Could you check a few things on this model? Use its own coordinates, in mm. Face numbers are marked on the shaded views. A direction names the side the tool comes from. Give positions to 0.01 mm unless a question says otherwise; leave off trailing zeros. Order: outer loops, then holes, each group sorted by start corner. A loop starts at its lowest first (then second) coordinate and runs counter-clockwise, first axis right, second up. Notation, with made-up numbers: M 10.25,70.5 L 39.25,70.5 A7 ccw 39.25,83.5 Z; hole C -5,60 d3. An arc over 180 degrees is marked long. Use a Markdown table: item, result. Add a question column.
```python
from build123d import *

# Parameters (mm, degrees)
F1_DEPTH = 21.59
F2_R     = 4.7625
F3_DEPTH = 25.4
F4_R     = 6.35
F5_DEPTH = 25.4
F6_R     = 10.16


with BuildPart() as f1:
    # F0 (on Top) → F1 (new body)
    with BuildSketch(Plane.XY):
        Polygon((53.34, 0), (0, 0), (-53.34, 0), (-65.4083, -34.193517), (-70.758128, -34.193517), (-68.58, -43.18), (-53.34, -43.18), (-43.478824, -15.24), (0, -15.24), (43.478824, -15.24), (53.34, -43.18), (68.58, -43.18), (70.758128, -34.193517), (65.4083, -34.193517), align=None)
    extrude(amount=F1_DEPTH)

    # F2 (on face) → F3 (cut)
    with BuildSketch(Plane.XZ.offset(43.18)):
        with Locations((-60.96, 10.795)):
            Circle(F2_R)
        with Locations((60.96, 10.795)):
            Circle(F2_R)
    extrude(amount=-F3_DEPTH, mode=Mode.SUBTRACT)

    # F4 (on face) → F5 (cut)
    with BuildSketch(Plane(origin=(0, 0, 0), x_dir=(-1, 0, 0), z_dir=(0, 1, 0))):
        with Locations((-61.568875, 10.795)):
            Circle(F4_R)
        with Locations((61.568875, 10.795)):
            Circle(F4_R)
    extrude(amount=-F5_DEPTH, mode=Mode.SUBTRACT)

    # F6
    f6_edges = [f1.edges().sort_by_distance(p)[0] for p in [
        (0, -15.24, 0),
        (48.409412, -29.21, 0),
        (-48.409412, -29.21, 0),
        (48.409412, -29.21, 21.59),
        (0, -15.24, 21.59),
        (-48.409412, -29.21, 21.59),
    ]]
    fillet(f6_edges, radius=F6_R)


solid = f1.part
```
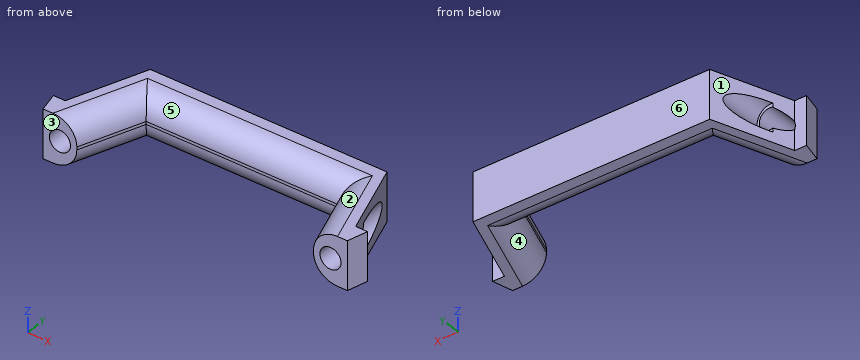
1) Suppose I cut it at D-D on z = 13.75. Please give me the cut outline in (x, y), and give its area (3 significant figures).
2) Suppose I cut it at B-B on x = -5. Please give me the cut outline in (y, z).
3) Suppose I cut it at A-A on z = 7.5. Please give me the cut outline in (x, y), and give its area (3 significant figures).
4) Suppose I cut it at C-C on z = 2.25. Please give me the cut outline in (x, y), and give its area (3 significant figures).
5) For pin 1 (4.5 mm diameter, centred on x = 68, z = 15.5, fed in from +Y); pin 2 (1 mm diameter, centred on x = 5, z = 11, fed in from -Y); pin 3 (11 mm diameter, centred on x = 60.96, z = 10.795, fed in from +Y), each with a flat end and sliding along its axis, tell me the tip position at first contact or that it passes through.
6) For the marked faces 4, 5 and 6, which set-ups out of +Z, -Z, +X, -X, +Y, -Y let a thin tool reach every point of the face, with its end or its side?
7) We'd pull the mould along X, two halves only. Please class the marked faces 1, 2 and 3: pulls with the +X half, pulls with the -X half, needs draft (parallel to the pull), parting line crosses it, or undercut.
8) Please list where these lines run through material, in increasing order: line 1 (Z direction, x = 60.96, y = -35.5); line 2 (Y direction, x = 21.5, z = 11); line 3 (X direction, y = -12.5, z = 11.25). Write a range as from..to.
Values found:
| question | item | result |
|---|---|---|
| 1 | outline | M -70.76,-34.19 L -68.58,-43.18 L -64.69,-43.18 L -64.69,-32.17 L -65.41,-34.19 Z; M -57.23,-43.18 L -53.62,-43.18 L -43.67,-14.97 L 43.67,-14.97 L 53.62,-43.18 L 57.23,-43.18 L 57.23,-25.4 L 55.95,-25.4 L 55.95,-7.39 L 53.34,0 L -53.34,0 L -55.95,-7.39 L -55.95,-25.4 L -57.23,-25.4 Z; M 64.69,-43.18 L 68.58,-43.18 L 70.76,-34.19 L 65.41,-34.19 L 64.69,-32.17 Z |
| 1 | area | 2,200 mm^2 |
| 2 | outline | M -15.24,10.16 A10.16 ccw -5.08,0 L 0,0 L 0,21.59 L -5.08,21.59 A10.16 ccw -15.24,11.43 Z |
| 3 | outline | M -70.76,-34.19 L -68.58,-43.18 L -64.4,-43.18 L -64.4,-31.33 L -65.41,-34.19 Z; M -57.52,-43.18 L -53.72,-43.18 L -43.73,-14.89 L 43.73,-14.89 L 53.72,-43.18 L 57.52,-43.18 L 57.52,-25.4 L 56.14,-25.4 L 56.14,-7.94 L 53.34,0 L -53.34,0 L -56.14,-7.94 L -56.14,-25.4 L -57.52,-25.4 Z; M 64.4,-43.18 L 68.58,-43.18 L 70.76,-34.19 L 65.41,-34.19 L 64.4,-31.33 Z |
| 3 | area | 2,220 mm^2 |
| 4 | outline | M -70.76,-34.19 L -68.58,-43.18 L -57.35,-43.18 L -46.16,-11.46 L 46.16,-11.46 L 57.35,-43.18 L 68.58,-43.18 L 70.76,-34.19 L 65.41,-34.19 L 53.34,0 L -53.34,0 L -65.41,-34.19 Z |
| 4 | area | 2,030 mm^2 |
| 5 | pin 1 | stops at y = -34.19 |
| 5 | pin 2 | stops at y = -15.24 |
| 5 | pin 3 | stops at y = -25.4 |
| 6 | face 4 | -Z, -Y |
| 6 | face 5 | +Z, -Y |
| 6 | face 6 | +Z, -Z, +X, -X, +Y |
| 7 | face 1 | pulls with the -X half |
| 7 | face 2 | undercut |
| 7 | face 3 | needs draft |
| 8 | line 1 | z = 0.01..6.03, 15.56..21.58 |
| 8 | line 2 | y = -15.24..0 |
| 8 | line 3 | x = -55.24..55.24 |
